Design review of the part built by this model. Coordinates are the model's own, in mm. Coordinates: 2 decimals unless noted, no trailing zeros. Order: outer loops, then holes, each group sorted by start corner. A loop starts at its lowest first (then second) coordinate and runs counter-clockwise, first axis right, second up. Notation, with made-up numbers: M 76.5,-32.5 L 89.5,-32.5 A21 cw 89.5,-20.5 Z; hole C -38.5,31 d8. An arc over 180 degrees is marked long. Use CSV: the item, a comma, the result in double quotes.
Autodesk Inventor part; units mm, degrees
ref_plane "YZ Plane" through (0, 0, 0) normal (1, 0, 0) x (0, 1, 0)
ref_plane "XZ Plane" through (0, 0, 0) normal (0, 1, 0) x (-1, 0, 0)
ref_plane "XY Plane" through (0, 0, 0) normal (0, 0, 1) x (1, 0, 0)
sketch "Sketch1" plane through (0, 0, 0) normal (0, 1, 0) x (-1, 0, 0)
  line L0 (101.6, 101.6) -> (-101.6, 101.6)
  line L1 (-101.6, 101.6) -> (-101.6, -101.6)
  line L2 (-101.6, -101.6) -> (101.6, -101.6)
  line L3 (101.6, -101.6) -> (101.6, 101.6)
  circle A0 centre (81.28, 85.725) radius 6.35
  circle A1 centre (81.28, -9.525) radius 6.35
  circle A2 centre (-82.55, 47.625) radius 6.35
  circle A3 centre (53.1707, -57.15) radius 4.953
  circle A4 centre (-2.7093, -57.15) radius 4.953
  circle A5 centre (87.376, 47.625) radius 4.953
  circle A6 centre (30.226, 47.625) radius 4.953
  point P0 (0, 0)
  dimension "d0" = 203.2
  dimension "d1" = 203.2
  dimension "d2" = 12.7
  dimension "d3" = 15.875
  dimension "d4" = 20.32
  dimension "d6" = 95.25
  dimension "d7" = 12.7
  dimension "d8" = 19.05
  dimension "d9" = 53.975
  dimension "d10" = 9.906
  dimension "d11" = 44.45
  dimension "d12" = 55.88
  dimension "d13" = 9.906
  dimension "d14" = 9.906
  dimension "d15" = 14.224
  dimension "d16" = 9.906
  dimension "d17" = 57.15
extrude "Extrusion1" add sketch "Sketch1" along normal blind 6.35
fillet "Fillet1" radius 6.35 4 edges at (-101.6, 3.175, 101.6) (101.6, 3.175, 101.6) (101.6, 3.175, -101.6) (-101.6, 3.175, -101.6)
properties part number "Nissan_Moter_Mount_Passenger"
(1) Add section A-A on z = -57.15. State the section outline as (x, y) points, and give its area (3 significant figures).
The answers:
outline,"M -101.6,0 L -58.12,0 L -58.12,6.35 L -101.6,6.35 Z; M -48.22,0 L -2.24,0 L -2.24,6.35 L -48.22,6.35 Z; M 7.66,0 L 101.6,0 L 101.6,6.35 L 7.66,6.35 Z"
area,"1,160 mm2"
(2) The part is to be moulded in two halves that separate along Z. For faces 1 (the face through (88.894, 3.131, 47.346)), 2 (the face through (-101.6, 3, -1)), 3 (the face through (1, 3, -101.6)), 4 (the face through (-99.79, 3.22, 99.69)), say which applies: pulls with the +Z half, pulls with the -Z half, needs draft (parallel to the pull), parting line crosses it, or undercut.
The answers:
face 1,"undercut"
face 2,"needs draft"
face 3,"pulls with the -Z half"
face 4,"pulls with the +Z half"
(3) Add section C-C on y = 4.5. State the section outline as (x, z) points (3 decimals).
The answers:
outline,"M -101.6,-95.25 A6.35 ccw -95.25,-101.6 L 95.25,-101.6 A6.35 ccw 101.6,-95.25 L 101.6,95.25 A6.35 ccw 95.25,101.6 L -95.25,101.6 A6.35 ccw -101.6,95.25 Z; hole C -87.376,47.625 d9.906; hole C -81.28,-9.525 d12.7; hole C -81.28,85.725 d12.7; hole C -53.171,-57.15 d9.906; hole C -30.226,47.625 d9.906; hole C 2.709,-57.15 d9.906; hole C 82.55,47.625 d12.7"
(4) Add section B-B on x = 82.55. State the section outline as (y, z) points (3 decimals).
The answers:
outline,"M 0,-101.6 L 6.35,-101.6 L 6.35,41.275 L 0,41.275 Z; M 0,53.975 L 6.35,53.975 L 6.35,101.6 L 0,101.6 Z"
(5) Wall thickness on probe 1 along Z at (x, y) = (-81.28, 2.25) (3 decimals); probe 2 along Z at (x, y) = (-30.5, 0.75); probe 3 along Z at (x, y) = (-49, 3.25): over which ranges is each line inside the solid? List them lowest first.
The answers:
probe 1,"z = -101.6 to -15.875, -3.175 to 79.375, 92.075 to 101.6"
probe 2,"z = -101.6 to 42.68, 52.57 to 101.6"
probe 3,"z = -101.6 to -59.82, -54.48 to 101.6"
